Verification items for the finished model (mm, model axes). A direction names the side the tool comes from. Give positions to 0.01 mm unless a question says otherwise; leave off trailing zeros. Loops run counter-clockwise (first coordinate to the right, second up) from the corner with the lowest first, then second, coordinate; pieces in that order, holes last. Notation, with made-up numbers: (60.5, 2) - (75.5, 2) arc R26 cw to (75.5, 23) - close; hole circle Ø2 at (33.25, 40.25). An arc over 180 degrees is marked (long way). One line per item, written item: value. Start each with the question number.
1. Scan lines: L1, parallel to Z at x = -0.5, y = -0.75; L2, parallel to X at y = -4.75, z = 5.5; L3, parallel to Y at x = 5, z = 16.5. Record each from-to range of solid material in increasing order. Write a range as [from, to].
2. Sectioned sample at D-D (y = -4). Record the cut outline in (x, z).
3. Mould release check, pull along X, two halves, no side actions. Record for faces 4 (the flat face through (-1, -5, 10)), 5 (the flat face through (10, 0, 10)), 6 (the flat face through (-2, 0, 6)): pulls with the +X half, pulls with the -X half, needs draft (parallel to the pull), parting line crosses it, or undercut.
4. Sectioned sample at C-C (z = 10). Record the cut outline in (x, y).
5. Sectioned sample at A-A (y = -1.25). Record the cut outline in (x, z).
6. Sectioned sample at B-B (z = 17). Record the cut outline in (x, y).
7. Gauge pin test, flat ends, axial feed: pin 1 (8 mm diameter, centred on x = 14.5, z = 4.5, fed in from -Y); pin 2 (3 mm diameter, centred on x = -2, y = -1.5, fed in from -Z); pin 3 (6.5 mm diameter, centred on y = 2, z = 4.5, fed in from -X). Record the tip position at first contact, or that the pin passes through.
8. Access from +Z, -Z, +X, -X, +Y, -Y to the whole of each face (thin tool, end or side, straight path). Record for faces 1 (the flat face through (8, 1, 20)), 2 (the flat face through (0, 0, 3)), 3 (the flat face through (-2, 0, 14)).
from build123d import *

# Parameters (mm, degrees)
F0_W      = 40
F0_H      = 10
F1_DEPTH  = 20
F3_DEPTH  = 20.001
F4_R      = 7.5
F5_DEPTH  = 10
F7_DEPTH  = 25
F8_DEPTH  = 20.001
F10_DEPTH = 10.001


with BuildPart() as f1:
    # F0 (on Top) → F1 (new body)
    with BuildSketch(Plane.XY):
        Rectangle(F0_W, F0_H)
    extrude(amount=F1_DEPTH)

    # F2 (on face) → F3 (cut, through all)
    with BuildSketch(Plane.XY.offset(20)):
        Polygon((20, -5), (20, 5), (0, -5), align=None)
    extrude(amount=-F3_DEPTH, mode=Mode.SUBTRACT)

    # F4 (on face) → F5 (join)
    with BuildSketch(Plane.XZ.offset(5)):
        with Locations((-10, 10)):
            Circle(F4_R)
    extrude(amount=F5_DEPTH)

    # F6 (on Top) → F7 (cut)
    with BuildSketch(Plane.XY):
        Polygon((-2.5, -15), (-17.5, -10), (-17.5, -15), align=None)
    extrude(amount=F7_DEPTH, mode=Mode.SUBTRACT)

    # F6 (on Top) → F8 (cut, through all)
    with BuildSketch(Plane.XY):
        Polygon((-2.5, -15), (-17.5, -10), (-17.5, -15), align=None)
    extrude(amount=F8_DEPTH, mode=Mode.SUBTRACT)

    # F9 (on face) → F10 (cut, through all)
    with BuildSketch(Plane.XZ.offset(5)):
        with BuildLine():
            Line((-3.655711, 14), (0, 14))
            Line((0, 14), (0, 20))
            Line((0, 20), (-20, 20))
            Line((-20, 20), (-20, 0))
            Line((-20, 0), (0, 0))
            Line((0, 0), (0, 6))
            Line((0, 6), (-3.655711, 6))
            ThreePointArc((-3.655711, 6), (-17.5, 10), (-3.655711, 14))
        make_face()
    extrude(amount=-F10_DEPTH, mode=Mode.SUBTRACT)


solid = f1.part
Results are:
1. L1: z = [6, 14]
1. L2: x = [-16, -4], [0, 0.5]
1. L3: y = [-2.5, 5]
2. outline: (-3.66, 6) - (0, 6) - (0, 0) - (2, 0) - (2, 20) - (0, 20) - (0, 14) - (-3.66, 14) arc R7.5 ccw (long way) to start
3. face 4: needs draft
3. face 5: pulls with the +X half
3. face 6: undercut
4. outline: (-17.5, -10) - (-2.5, -15) - (-2.5, -5) - (0, -5) - (20, 5) - (-17.5, 5) - close
5. outline: (-3.66, 6) - (0, 6) - (0, 0) - (7.5, 0) - (7.5, 20) - (0, 20) - (0, 14) - (-3.66, 14) arc R7.5 ccw (long way) to start
6. outline: (-12.69, -11.6) - (-7.31, -13.4) - (-7.31, 5) - (-12.69, 5) - close; (0, -5) - (20, 5) - (0, 5) - close
7. pin 1: stops at y = 0.25
7. pin 2: stops at z = 6
7. pin 3: stops at x = -17.15
8. face 1: +Z, +X, -X, +Y, -Y
8. face 2: -Z, +Y, -Y
8. face 3: +Z, +Y, -Y
